Read the model definition and answer for the solid it produces. Units are mm, in the model's axes. Coordinates: 2 decimals unless noted, no trailing zeros. Loops run counter-clockwise (first coordinate to the right, second up) from the corner with the lowest first, then second, coordinate; pieces in that order, holes last.
from build123d import *

# Parameters (mm, degrees)
ESQUISSE1_R             = 32.5
BOSS_EXTRU_1_DEPTH      = 18
ESQUISSE3_R             = 1.5
ENL_V_MAT_EXTRU_1_DEPTH = 3
ESQUISSE4_R             = 14.75
BOSS_EXTRU_3_DEPTH      = 12


with BuildPart() as part:
    # Esquisse1 → Boss.-Extru.1 (new body)
    with BuildSketch(Plane(origin=(0, 0, 0), x_dir=(1, 0, 0), z_dir=(0, 1, 0))):
        Circle(ESQUISSE1_R)
    extrude(amount=BOSS_EXTRU_1_DEPTH)

    # Esquisse2 → Enlèvement de matière-Révolution1 (revolve, cut)
    with BuildSketch(Plane.XY):
        with BuildLine():
            Line((-32.5, 13), (-32.5, 19))
            Line((-32.5, 19), (0, 19))
            Line((0, 19), (0, 18))
            add(Edge.make_bspline(
                [(-32.5, 13), (-32.5, 14.172258114), (-21.601405785, 18), (0, 18)],
                knots=[0, 0, 0, 0, 1, 1, 1, 1], degree=3))
        make_face()
    revolve(axis=Axis((0, 0, 0), (0, 1, 0)), mode=Mode.SUBTRACT)

    # Esquisse3 → Enlèv. mat.-Extru.1 (cut)
    with BuildSketch(Plane(origin=(0, 18, 0), x_dir=(1, 0, 0), z_dir=(0, 1, 0))):
        with Locations((-18.384776311, -18.384776311)):
            Circle(ESQUISSE3_R)
    extrude(amount=-ENL_V_MAT_EXTRU_1_DEPTH, mode=Mode.SUBTRACT)

    # Esquisse4 → Boss.-Extru.3 (add)
    with BuildSketch(Plane(origin=(0, 0, 0), x_dir=(1, 0, 0), z_dir=(0, 1, 0))):
        Circle(ESQUISSE4_R)
    extrude(amount=-BOSS_EXTRU_3_DEPTH)


solid = part.part
Q1. Flat-ended cylindrical pins translate along their axes: pin 1 Ø2.5 at (x, z) = (-18, 18.5) entering from +Y; pin 2 Ø1.5 at (x, y) = (-12.5, -5) entering from -Z; pin 3 Ø4 at (x, z) = (16.5, 7.5) entering from +Y. Find the tip coordinate at first contact, or state that the pin passes through.
Findings below:
pin 1: stops at y = 15.9
pin 2: stops at z = -8.92
pin 3: stops at y = 17.19
Q2. Straight lines are drawn through the part: probe 1 along Y at (x, z) = (1, 0.5); probe 2 along Y at (x, z) = (-10, 8); probe 3 along X at (y, z) = (-7.5, -13). For each, find the intervals that lie inside material, in ascending order.
Findings below:
probe 1: y = -12 to 18
probe 2: y = -12 to 17.5
probe 3: x = -6.97 to 6.97
Q3. A cutting plane is placed at A-A (y = -1). Give the vertices of the cut face in (x, z), then the cut area to 3 significant figures.
Findings below:
outline: circle Ø29.5 at (0, 0)
area: 683 mm2
Q4. A cutting plane is placed at B-B (y = 8). Give the vertices of the cut face in (x, z).
Findings below:
outline: circle Ø65 at (0, 0)
Q5. Determine the mould class of faces 1 (the face through (-18, 15, 18)), 2 (the face through (-17.58, 15.36, 17.12)), 3 (the face through (14, 0, 7)), 4 (the face through (14.07, -5.92, -4.43)) for opening direction Z: +Z half, -Z half, draft (parallel to the pull), parting line (faces both ways), or undercut.
Findings below:
face 1: undercut
face 2: undercut
face 3: draft
face 4: parting line
